from build123d import *

# Parameters (mm, degrees)
SKETCH1_R           = 50.1
SKETCH1_W           = 40.4
SKETCH1_H           = 40.4
BOSS_EXTRUDE1_DEPTH = 13
SKETCH4_W           = 4.5
SKETCH4_H           = 19
SKETCH4_W_2         = 19
SKETCH4_H_2         = 4.5
CUT_EXTRUDE1_DEPTH  = 1.5
SKETCH5_W           = 4.5
SKETCH5_H           = 19
SKETCH5_W_2         = 19
SKETCH5_H_2         = 4.5
CUT_EXTRUDE2_DEPTH  = 1.5
SKETCH6_R           = 1.975
CUT_EXTRUDE3_DEPTH  = 21.5
SKETCH8_R           = 1.975
CUT_EXTRUDE4_DEPTH  = 21.5
CUT_EXTRUDE5_DEPTH  = 3.7
CUT_EXTRUDE6_DEPTH  = 3.7
CUT_EXTRUDE7_START  = -24
SKETCH11_R          = 50.1
SKETCH11_R_2        = 47.6
CUT_EXTRUDE7_DEPTH  = 24
SKETCH12_R          = 47.65
SKETCH12_R_2        = 47.6
BOSS_EXTRUDE2_DEPTH = 13


with BuildPart() as part:
    # Sketch1 → Boss-Extrude1 (new body)
    with BuildSketch(Plane(origin=(0, 0, 0), x_dir=(1, 0, 0), z_dir=(0, 1, 0))):
        with Locations(Location((0, 0, 0), (0, 0, 90))):
            Circle(SKETCH1_R)
        Rectangle(SKETCH1_W, SKETCH1_H, mode=Mode.SUBTRACT)
    extrude(amount=BOSS_EXTRUDE1_DEPTH)

    # Sketch4 → Cut-Extrude1 (cut)
    with BuildSketch(Plane(origin=(0, 13, 0), x_dir=(1, 0, 0), z_dir=(0, 1, 0))):
        with Locations((-10.2, 29.7)):
            Rectangle(SKETCH4_W, SKETCH4_H)
        with Locations((29.7, -10.2)):
            Rectangle(SKETCH4_W_2, SKETCH4_H_2)
        with Locations((10.2, -29.7)):
            Rectangle(SKETCH4_W, SKETCH4_H)
        with Locations((-29.7, 10.2)):
            Rectangle(SKETCH4_W_2, SKETCH4_H_2)
    extrude(amount=-CUT_EXTRUDE1_DEPTH, mode=Mode.SUBTRACT)

    # Sketch5 → Cut-Extrude2 (cut)
    with BuildSketch(Plane.XZ):
        with Locations((-10.2, 29.7)):
            Rectangle(SKETCH5_W, SKETCH5_H)
        with Locations((29.7, -10.2)):
            Rectangle(SKETCH5_W_2, SKETCH5_H_2)
        with Locations((10.2, -29.7)):
            Rectangle(SKETCH5_W, SKETCH5_H)
        with Locations((-29.7, 10.2)):
            Rectangle(SKETCH5_W_2, SKETCH5_H_2)
    extrude(amount=-CUT_EXTRUDE2_DEPTH, mode=Mode.SUBTRACT)

    # Sketch6 → Cut-Extrude3 (cut)
    with BuildSketch(Plane(origin=(0, 13, 0), x_dir=(1, 0, 0), z_dir=(0, 1, 0))):
        with Locations(Location((31.925, -10.2, 0), (0, 0, 270))):
            Circle(SKETCH6_R)
        with Locations(Location((-10.2, 31.925, 0), (0, 0, 270))):
            Circle(SKETCH6_R)
        with Locations(Location((-31.925, 10.2, 0), (0, 0, 270))):
            Circle(SKETCH6_R)
        with Locations(Location((10.2, -31.925, 0), (0, 0, 270))):
            Circle(SKETCH6_R)
    extrude(amount=-CUT_EXTRUDE3_DEPTH, mode=Mode.SUBTRACT)

    # Sketch8 → Cut-Extrude4 (cut)
    with BuildSketch(Plane.XZ):
        with Locations(Location((-10.2, 31.925, 0), (0, 0, 90))):
            Circle(SKETCH8_R)
        with Locations(Location((31.925, -10.2, 0), (0, 0, 270))):
            Circle(SKETCH8_R)
        with Locations(Location((10.2, -31.925, 0), (0, 0, 270))):
            Circle(SKETCH8_R)
        with Locations(Location((-31.925, 10.2, 0), (0, 0, 270))):
            Circle(SKETCH8_R)
    extrude(amount=-CUT_EXTRUDE4_DEPTH, mode=Mode.SUBTRACT)

    # Sketch9 → Cut-Extrude5 (cut)
    with BuildSketch(Plane.XZ):
        Polygon((14.530127019, 31.925), (12.365063509, 35.675), (8.034936491, 35.675), (5.869872981, 31.925), (8.034936491, 28.175), (12.365063509, 28.175), align=None)
        Polygon((36.255127019, 10.2), (34.090063509, 13.95), (29.759936491, 13.95), (27.594872981, 10.2), (29.759936491, 6.45), (34.090063509, 6.45), align=None)
        Polygon((-27.594872981, -10.2), (-29.759936491, -6.45), (-34.090063509, -6.45), (-36.255127019, -10.2), (-34.090063509, -13.95), (-29.759936491, -13.95), align=None)
        Polygon((-5.869872981, -31.925), (-8.034936491, -28.175), (-12.365063509, -28.175), (-14.530127019, -31.925), (-12.365063509, -35.675), (-8.034936491, -35.675), align=None)
    extrude(amount=-CUT_EXTRUDE5_DEPTH, mode=Mode.SUBTRACT)

    # Sketch10 → Cut-Extrude6 (cut)
    with BuildSketch(Plane(origin=(0, 13, 0), x_dir=(1, 0, 0), z_dir=(0, 1, 0))):
        Polygon((14.530127019, 31.925), (12.365063509, 35.675), (8.034936491, 35.675), (5.869872981, 31.925), (8.034936491, 28.175), (12.365063509, 28.175), align=None)
        Polygon((36.255127019, 10.2), (34.090063509, 13.95), (29.759936491, 13.95), (27.594872981, 10.2), (29.759936491, 6.45), (34.090063509, 6.45), align=None)
        Polygon((-5.869872981, -31.925), (-8.034936491, -28.175), (-12.365063509, -28.175), (-14.530127019, -31.925), (-12.365063509, -35.675), (-8.034936491, -35.675), align=None)
        Polygon((-27.594872981, -10.2), (-29.759936491, -6.45), (-34.090063509, -6.45), (-36.255127019, -10.2), (-34.090063509, -13.95), (-29.759936491, -13.95), align=None)
    extrude(amount=-CUT_EXTRUDE6_DEPTH, mode=Mode.SUBTRACT)

    # Sketch11 → Cut-Extrude7 (cut)
    with BuildSketch(Plane(origin=(0, 13, 0), x_dir=(1, 0, 0), z_dir=(0, 1, 0)).offset(CUT_EXTRUDE7_START)):
        Circle(SKETCH11_R)
        with Locations(Location((0, 0, 0), (0, 0, 270))):
            Circle(SKETCH11_R_2, mode=Mode.SUBTRACT)
    extrude(amount=CUT_EXTRUDE7_DEPTH, mode=Mode.SUBTRACT)

    # Sketch12 → Boss-Extrude2 (add)
    with BuildSketch(Plane.XZ):
        with Locations(Location((0, 0, 0), (0, 0, 270))):
            Circle(SKETCH12_R)
        Circle(SKETCH12_R_2, mode=Mode.SUBTRACT)
    extrude(amount=-BOSS_EXTRUDE2_DEPTH)


solid = part.part
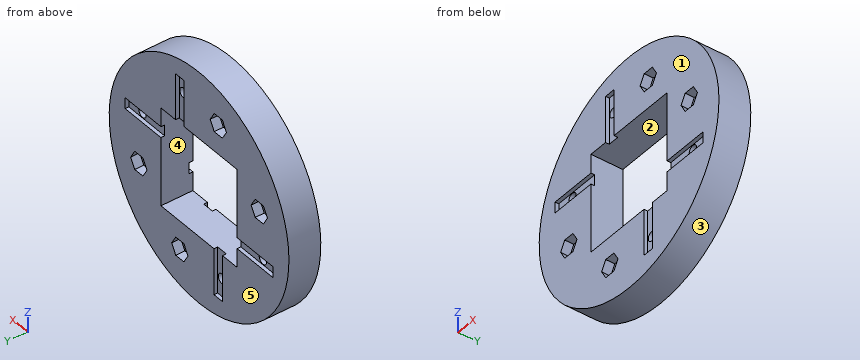
Verification items for the finished model (mm, model axes). Face numbers are marked on the shaded views. A direction names the side the tool comes from. Give positions to 0.01 mm unless a question says otherwise; leave off trailing zeros. Loops run counter-clockwise (first coordinate to the right, second up) from the corner with the lowest first, then second, coordinate; pieces in that order, holes last.
1) Sectioned sample at B-B, the plane x = 0. Enter the section's corners in (y, z).
2) Set-up check for the marked faces 1 and 2: record each of +Z, -Z, +X, -X, +Y, -Y from which the full face is reachable in a straight line by a thin tool's end or side.
3) Sectioned sample at D-D, the plane x = 10.2. Enter the section's corners in (y, z) (3 decimals).
4) Sectioned sample at A-A, the plane z = 0. Enter the section's corners in (x, y), then the cut area to 3 significant figures.
5) Sectioned sample at C-C, the plane y = 6.5. Count the separate pieces of the cut face and the enclosed holes in it, then the cut area to 3 significant figures.
6) Depth check by flat-ended pin: pin 1 Ø1.2 at (y, z) = (0.5, -10) entering from -X; pin 2 Ø3.5 at (x, z) = (-30, -10) entering from +Y; pin 3 Ø6.5 at (x, z) = (10.2, -31.925) entering from +Y; pin 4 Ø2.5 at (x, z) = (10.2, 31.925) entering from +Y. Enter the tip coordinate at first touch or a pass-through.
7) Draft check along Z on the marked faces 3, 4 and 5. Enter one of: pulls with the +Z half, pulls with the -Z half, needs draft (parallel to the pull), parting line crosses it, or undercut.
8) Thickness scan on line 1 along Z through (x, y) = (-1.5, 1.25); line 2 along X through (y, z) = (12, -29); line 3 along X through (y, z) = (4.5, -31) (3 decimals). Record the ranges inside material, lowest first.
Answers:
1. outline: (0, -47.65) - (13, -47.65) - (13, -20.2) - (0, -20.2) - close; (0, 20.2) - (13, 20.2) - (13, 47.65) - (0, 47.65) - close
2. face 1: +Z, -Z, +X, -X, -Y
2. face 2: +Y, -Y
3. outline: (0, -46.545) - (13, -46.545) - (13, -35.675) - (9.3, -35.675) - (9.3, -33.9) - (1.5, -33.9) - (1.5, -39.2) - (0, -39.2) - close; (0, 20.2) - (11.5, 20.2) - (11.5, 29.95) - (3.7, 29.95) - (3.7, 28.175) - (0, 28.175) - close; (0, 35.675) - (3.7, 35.675) - (3.7, 33.9) - (11.5, 33.9) - (11.5, 39.2) - (13, 39.2) - (13, 46.545) - (0, 46.545) - close; (1.5, -29.95) - (9.3, -29.95) - (9.3, -28.175) - (13, -28.175) - (13, -20.2) - (1.5, -20.2) - close
4. outline: (-47.65, 0) - (-20.2, 0) - (-20.2, 13) - (-47.65, 13) - close; (20.2, 0) - (47.65, 0) - (47.65, 13) - (20.2, 13) - close
4. area: 714 mm2
5. separate pieces: 1
5. enclosed holes: 9
5. area: 5,400 mm2
6. pin 1: stops at x = -46.71
6. pin 2: stops at y = 11.5
6. pin 3: stops at y = 9.3
6. pin 4: passes through
7. face 3: parting line crosses it
7. face 4: undercut
7. face 5: needs draft
8. line 1: z = -47.63 to -20.2, 20.2 to 47.63
8. line 2: x = -37.81 to -12.45, -7.95 to 7.56, 12.84 to 37.81
8. line 3: x = -36.187 to -11.945, -8.455 to 8.455, 11.945 to 36.187
